Part model, mm, in its own coordinate system. Round coordinates to 2 decimals unless told otherwise and drop trailing zeros. Write each loop counter-clockwise with the first axis right and the second up, starting at its lowest first coordinate (ties: lowest second). Pieces come first, ordered by that corner, then holes. Notation, with made-up numbers: M 8.5,54 L 40.5,54 A28 ccw 40.5,93 Z; hole C 10.5,-26.5 d11. An arc over 180 degrees is marked long. Answer as a JSON object with one key per item and string values. Group by question number.
1. Band-saw the part on B-B, the plane y = 452. Write the cut outline in (x, z), plus the area to 3 significant figures.
2. Drill centre lines: line 1 (Y direction, x = 0, z = 0.65) (3 decimals); line 2 (X direction, y = 220, z = 0.5); line 3 (X direction, y = 304.5, z = 1.5). Where is each one in solid material? Low to high. Write a range as from..to.
3. Band-saw the part on A-A, the plane x = -3.25. Write the cut outline in (y, z), plus the area to 3 significant figures.
4. Drop flat-ended pins along their axis: pin 1 (1.5 mm diameter, centred on y = 286, z = 1.5, fed in from +X); pin 2 (3 mm diameter, centred on x = 0, y = 495.435, fed in from -Z); pin 3 (1.5 mm diameter, centred on x = -3.5, y = 435, fed in from +Z); pin 4 (1.8 mm diameter, centred on x = 0, y = 4.565, fed in from -Z). Give the stop position or say it passes through.
Autodesk Inventor part; units mm, degrees
ref_plane "Work Plane1" through (5, 0, 0) normal (1, 0, 0) x (0, 1, 0)
ref_plane "Work Plane2" through (0, 250, 0) normal (0, -1, 0) x (1, 0, 0)
ref_plane "XZ Plane" through (0, 0, 0) normal (0, 1, 0) x (-1, 0, 0)
sketch "Sketch1" plane through (0, 0, 0) normal (0, 1, 0) x (-1, 0, 0)
  circle A0 centre (0, 0) radius 5
  dimension "d0" = 10
extrude "Extrusion1" add sketch "Sketch1" along normal blind 500
ref_plane "Work Plane1" through (5, 0, 0) normal (1, 0, 0) x (0, 1, 0)
sketch "Sketch2" plane through (5, 0, 0) normal (1, 0, 0) x (0, 1, 0)
  line L0 (500, -5) -> (500, 5)
  line L1 (0, 5) -> (0, -5)
  line L2 (0, 5) -> (500, 5)
  line L3 (0, -5) -> (500, -5)
  line L4 (0, 0) -> (0, 1.5)
  line L5 (0, 5) -> (0, -5)
  line L6 (0, 0) -> (0, -1.5)
  line L7 (-100, 0) -> (600, 0)
  line L8 (0, 1.5) -> (20, 5)
  line L9 (20, 5) -> (20, -5)
  line L10 (20, -5) -> (0, -1.5)
  dimension "d4" = 1.5
  dimension "d5" = 1.5
  dimension "d6" = 20
extrude "Extrusion2" cut sketch "Sketch2" against normal blind 500 contours L3 L1 L10 | L8 L1 L2
sketch "Sketch3" plane through (0, 0, 0) normal (0, 0, 1) x (1, 0, 0)
  point P0 (0, 0)
sketch "Sketch4" plane through (0, 0, 0) normal (0, 0, 1) x (1, 0, 0)
  circle A0 centre (0, 4.565) radius 1
  point P0 (0, 0)
  dimension "d9" = 2
extrude "Extrusion3" cut sketch "Sketch4" along normal mid plane 500
ref_plane "Work Plane2" through (0, 250, 0) normal (0, -1, 0) x (1, 0, 0)
mirror "Mirror1" about plane through (0, 250, 0) normal (0, -1, 0) of "Extrusion2", "Extrusion3"
properties part number "Straight connector"
Worked answers:
{
 "1": {"outline": "C 0,0 d10", "area": "78.5 mm^2"},
 "2": {"line 1": "y = 0..3.565, 5.565..494.435, 496.435..500", "line 2": "x = -4.97..4.97", "line 3": "x = -4.77..4.77"},
 "3": {"outline": "M 0,-1.5 L 13.14,-3.8 L 486.86,-3.8 L 500,-1.5 L 500,1.5 L 486.86,3.8 L 13.14,3.8 L 0,1.5 Z", "area": "3,740 mm^2"},
 "4": {"pin 1": "stops at x = 4.94", "pin 2": "stops at z = -2.56", "pin 3": "stops at z = 4.18", "pin 4": "passes through"}
}
